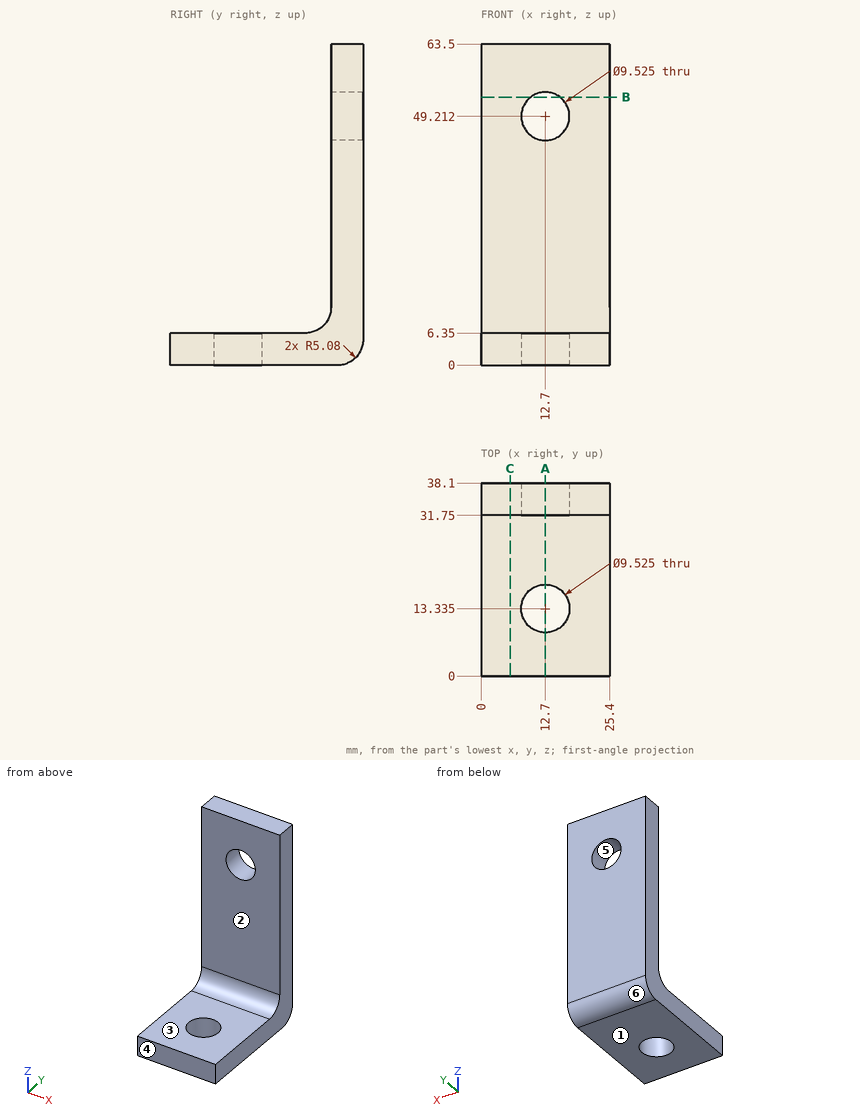
The drawing under review shows one solid part. Ordinate dimensions are in mm from its lowest x, y, z. A direction names the side the tool comes from. Round coordinates to 2 decimals unless told otherwise and drop trailing zeros. Write each loop counter-clockwise with the first axis right and the second up, starting at its lowest first coordinate (ties: lowest second). Pieces come first, ordered by that corner, then holes. Notation, with made-up numbers: (30, 57) -> (71, 57) arc R21 ccw to (71, 95) -> close; hole circle Ø7 at (79, 27.5). An arc over 180 degrees is marked (long way). One line per question, with ' | ' between items. Start each with the question number.
(1) Insertion check: P1, Ø12.5, axis at x = 15, z = 43, coming from the -Y side; P2, Ø8.5, axis at x = 12.7, z = 49.21, coming from the -Y side; P3, Ø3, axis at x = 7.5, y = 17.5, coming from the +Z side; P4, Ø6, axis at x = 13, y = 23, coming from the +Z side. Each pin has a flat end and moves straight along its axis. Give the tip position at first contact, or say it passes through.
(2) For line 1 along Z through (x, y) = (17, 4); line 2 along Y through (x, z) = (5.75, 35); line 3 along X through (y, z) = (12.5, 4), list the stretches that pass through material, from the lowest coordinate up. Write a range as from..to.
(3) Add section C-C, the plane x = 5.75. Write out the cut boundary in (y, z), plus the area to 3 significant figures.
(4) Mouldability with a two-part tool opening along Z and no side actions: class the marked faces 3, 4, 5 and 6 as released by +Z, released by -Z, zero draft, split by the parting line, or undercut.
(5) Add section B-B, the plane z = 53. Write out the cut boundary in (x, y), plus the area to 3 significant figures.
(6) Tool access review of the marked faces 1 and 2: name each direction out of +Z, -Z, +X, -X, +Y, -Y from which nothing blocks a thin tool from reaching the whole face with its end or side.
(7) Add section A-A, the plane x = 12.7. Give the number of separate pieces and of enclosed holes in the cut face, plus the area to 3 significant figures.
Answer list:
1) P1: y = 31.75 | P2: through | P3: z = 6.35 | P4: z = 6.35
2) line 1: 0..6.35 | line 2: 31.75..38.1 | line 3: 0..8.01, 17.39..25.4
3) outline: (0, 0) -> (33.02, 0) arc R5.08 ccw to (38.1, 5.08) -> (38.1, 63.5) -> (31.75, 63.5) -> (31.75, 11.43) arc R5.08 cw to (26.67, 6.35) -> (0, 6.35) -> close | area: 605 mm²
4) face 3: released by +Z | face 4: zero draft | face 5: undercut | face 6: released by -Z
5) outline: (0, 31.75) -> (9.81, 31.75) -> (9.81, 38.1) -> (0, 38.1) -> close; (15.59, 31.75) -> (25.4, 31.75) -> (25.4, 38.1) -> (15.59, 38.1) -> close | area: 125 mm²
6) face 1: -Z, +X, -X, +Y, -Y | face 2: +Z, +X, -X, -Y
7) separate pieces: 3 | enclosed holes: 0 | area: 484 mm²
